from build123d import *

# Parameters (mm, degrees)
F0_W           = 278.2998234034
F0_H           = 152.0985364914
F1_DEPTH       = 76.2
F3_D           = 16.51
F4_D           = 16.51
F4_DEPTH       = 12.7
F4_TIP         = 4.9601044101
F5_D           = 16.51
F5_DEPTH       = 12.7
F5_CBORE_D     = 19.05
F5_CBORE_DEPTH = 12.7
F5_TIP         = 4.9601044101
F6_D           = 15.24
F6_CSINK_D     = 19.05
F6_CSINK_ANGLE = 45
F7_D           = 15.24
F7_CSINK_D     = 19.05
F7_CSINK_ANGLE = 45


with BuildPart() as f1:
    # F0 (on Front) → F1 (new body)
    with BuildSketch(Plane.XZ):
        with Locations((2.0410194993, 1.6697347164)):
            Rectangle(F0_W, F0_H)
    extrude(amount=F1_DEPTH)

    # F3 (through all)
    with Locations(Plane.XZ.offset(76.2)):
        with Locations((-58.4882125258, 46.6711297631)):
            Hole(F3_D / 2)

    # F4
    with Locations(Plane.XZ.offset(76.2)):
        with Locations((-6.3315038569, 26.0829553008)):
            Hole(F4_D / 2, depth=F4_DEPTH)
            with Locations((0, 0, -(F4_DEPTH + F4_TIP / 2))):  # 118° drill point
                Cone(0, F4_D / 2, F4_TIP, mode=Mode.SUBTRACT)

    # F5
    with Locations(Plane.XZ.offset(76.2)):
        with Locations((32.0997536182, 48.455439508)):
            CounterBoreHole(F5_D / 2, F5_CBORE_D / 2, F5_CBORE_DEPTH, depth=F5_DEPTH)
            with Locations((0, 0, -(F5_DEPTH + F5_TIP / 2))):  # 118° drill point
                Cone(0, F5_D / 2, F5_TIP, mode=Mode.SUBTRACT)

    # F6 (through all)
    with Locations(Plane.XZ.offset(76.2)):
        with Locations((11.0998153687, -35.6815680861)):
            CounterSinkHole(F6_D / 2, F6_CSINK_D / 2, counter_sink_angle=F6_CSINK_ANGLE)

    # F7 (through all)
    with Locations(Plane.XZ.offset(76.2)):
        with Locations((135.4523897171, -71.9167515635), (47.6095117629, -47.8972196579), (58.315359056, -54.0736690164)):
            CounterSinkHole(F7_D / 2, F7_CSINK_D / 2, counter_sink_angle=F7_CSINK_ANGLE)


solid = f1.part
Here's how the part is built. I have some questions about the finished solid (model axes, mm). A direction names the side the tool comes from. Round coordinates to 2 decimals unless told otherwise and drop trailing zeros. Order: outer loops, then holes, each group sorted by start corner. A loop starts at its lowest first (then second) coordinate and runs counter-clockwise, first axis right, second up. Notation, with made-up numbers: (44, 52) -> (98, 52) arc R36 cw to (98, 89) -> close; hole circle Ø7 at (4, 1.25). An arc over 180 degrees is marked (long way). Use CSV: the item, a comma, the result in double quotes.
1. I want a section at A-A on y = -17. List the corners of the cut face in (x, z) for me (3 decimals), and give its area (3 significant figures).
Recorded:
outline,"(-137.109, -74.38) -> (128.241, -74.38) arc R7.62 cw to (141.191, -66.903) -> (141.191, 77.719) -> (-137.109, 77.719) -> close; hole circle Ø16.51 at (-58.488, 46.671); hole circle Ø15.24 at (11.1, -35.682); hole (50.735, -54.847) arc R7.62 ccw (long way) to (55.19, -47.124) arc R7.62 ccw (long way) to start"
area,"41,500 mm2"
2. Thinking about a two-plate mould opening in X: for faces 3 (the face through (141.191, -38, 4)), 4 (the face through (30.86, -69.94, 57.9)), 5 (the face through (0, 0, 3)), which applies, pulls with the +X half, pulls with the -X half, needs draft (parallel to the pull), parting line crosses it, or undercut?
Recorded:
face 3,"pulls with the +X half"
face 4,"undercut"
face 5,"needs draft"
3. I need wall thicknesses on line 1 along X through (y, z) = (-67.5, -41); line 2 along X through (y, z) = (-44, -30); line 3 along Z through (x, y) = (6, -19.5). Which ranges of each line are inside material? Lowest first, please.
Recorded:
line 1,"x = -137.11 to 5.64, 16.56 to 44.37, 50.85 to 141.19"
line 2,"x = -137.11 to 6.02, 16.18 to 141.19"
line 3,"z = -74.38 to -41.34, -30.02 to 77.72"
4. Which directions (+Z, -Z, +X, -X, +Y, -Y) give clear straight access to the entire face, cutting with the end or side of a thin tool? Please do faces 1 (the face through (25, -63.5, 53)), 2 (the face through (-66.114, -37.567, 43.509)).
Recorded:
face 1,"-Y"
face 2,"+Y, -Y"
5. I want a section at B-B on x = -56. List the corners of the cut face in (y, z) for me, and give its area (3 significant figures).
Recorded:
outline,"(-76.2, -74.38) -> (0, -74.38) -> (0, 38.8) -> (-76.2, 38.8) -> close; (-76.2, 54.54) -> (0, 54.54) -> (0, 77.72) -> (-76.2, 77.72) -> close"
area,"10,400 mm2"
